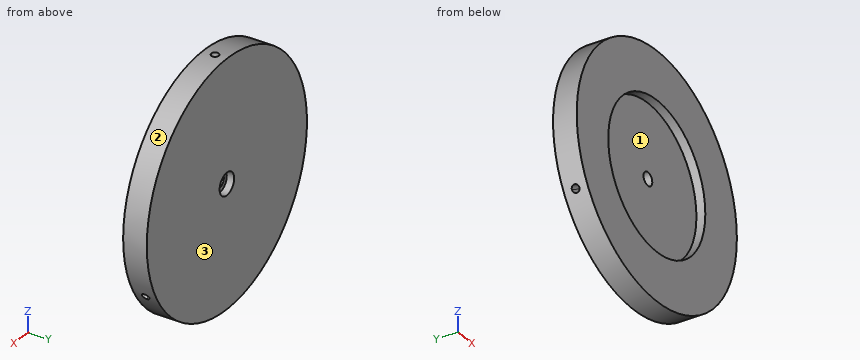
from build123d import *

# Parameters (mm, degrees)
F0_R            = 82.5
F1_DEPTH        = 16
F2_R            = 50
F3_DEPTH        = 6
F6_DEPTH        = 28
F6_COPIES_COUNT = 3
F7_R            = 4.5
F8_DEPTH        = 25
F9_R            = 7.5
F9_R_2          = 4.5
F10_DEPTH       = 5


# Not quite as in the source:
# - a pattern or mirror of a feature is missing from the dataset's text; its kind, count and spacing are read off the source's solid


with BuildPart() as f1:
    # F0 (on Front) → F1 (new body)
    with BuildSketch(Plane.XZ):
        Circle(F0_R)
    extrude(amount=F1_DEPTH)

    # F2 (on face) → F3 (cut)
    with BuildSketch(Plane.XZ.offset(16)):
        Circle(F2_R)
    extrude(amount=-F3_DEPTH, mode=Mode.SUBTRACT)

    # F5 (on offset) → F6 (cut)
    with BuildSketch(Plane.XY.offset(82.5)):
        with BuildLine():
            ThreePointArc((2.5, -8), (1.767766953, -6.232233047), (0, -5.5))
            Line((0, -5.5), (0, -10.5))
            ThreePointArc((0, -10.5), (1.767766953, -9.767766953), (2.5, -8))
        make_face()
        with BuildLine():
            Line((0, -10.5), (0, -5.5))
            ThreePointArc((0, -5.5), (-2.5, -8), (0, -10.5))
        make_face()
    f6 = extrude(amount=-F6_DEPTH, mode=Mode.SUBTRACT)

    # F6_copies: F6 ×3 about axis
    f6_copies_axis = Axis((0, 0, 0), (0, 1, 0))
    for i in range(1, F6_COPIES_COUNT):
        add(f6.rotate(f6_copies_axis, i * 360 / F6_COPIES_COUNT), mode=Mode.SUBTRACT)

    # F7 (on face) → F8 (cut)
    with BuildSketch(Plane.XZ.offset(10)):
        Circle(F7_R)
    extrude(amount=-F8_DEPTH, mode=Mode.SUBTRACT)

    # F9 (on face) → F10 (cut)
    with BuildSketch(Plane(origin=(0, 0, 0), x_dir=(-1, 0, 0), z_dir=(0, 1, 0))):
        Circle(F9_R)
        Circle(F9_R_2, mode=Mode.SUBTRACT)
    extrude(amount=-F10_DEPTH, mode=Mode.SUBTRACT)


solid = f1.part
Read the model definition and answer for the solid it produces. Units are mm, in the model's axes. Face numbers are marked on the shaded views. Round coordinates to 2 decimals unless told otherwise and drop trailing zeros. Order: outer loops, then holes, each group sorted by start corner. A loop starts at its lowest first (then second) coordinate and runs counter-clockwise, first axis right, second up.
1) Flat-ended cylindrical pins translate along their axes: pin 1 (8 mm diameter, centred on x = 38, z = -24, fed in from +Y); pin 2 (8 mm diameter, centred on x = 18, y = -12, fed in from +Z); pin 3 (7.5 mm diameter, centred on x = 2, z = 0.5, fed in from +Y); pin 4 (3 mm diameter, centred on x = 30, y = -12.5, fed in from +Z). Find the tip coordinate at first contact, or state that the pin passes through.
2) Straight lines are drawn through the part: L1, parallel to X at y = -15, z = -1; L2, parallel to Z at x = 0, y = -8.5; L3, parallel to Y at x = -23.5, z = -30.5. For each, find the intervals that lie inside material, in ascending order.
3) The part is cut by section B-B on x = -21. Write down the section's boundary in (y, z), plus the area to 3 significant figures.
4) The part is cut by section A-A on z = 0. Write down the section's boundary in (x, y).
5) The part is cut by section C-C on z = 67. Write down the section's boundary in (x, y), plus the area to 3 significant figures.
6) The part is cut by section D-D on z = 24.5. Write down the section's boundary in (x, y), plus the area to 3 significant figures.
7) The mould has two halves that part along Z. Classify the marked faces 1, 2 and 3: released by +Z, released by -Z, zero draft, split by the parting line, or undercut.
Resolved:
1. pin 1: stops at y = 0
1. pin 2: stops at z = 81.3
1. pin 3: stops at y = -5
1. pin 4: stops at z = 77.42
2. L1: x = -82.49 to -49.99, 49.99 to 82.49
2. L2: z = -82.5 to -4.5, 4.5 to 54.5
2. L3: y = -10 to 0
3. outline: (-16, -79.78) - (0, -79.78) - (0, 79.78) - (-16, 79.78) - (-16, 45.38) - (-10, 45.38) - (-10, -45.38) - (-16, -45.38) - close
3. area: 2,010 mm2
4. outline: (-82.5, -16) - (-50, -16) - (-50, -10) - (-4.5, -10) - (-4.5, -5) - (-7.5, -5) - (-7.5, 0) - (-82.5, 0) - close; (4.5, -10) - (50, -10) - (50, -16) - (82.5, -16) - (82.5, 0) - (7.5, 0) - (7.5, -5) - (4.5, -5) - close
5. outline: (-48.14, -16) - (48.14, -16) - (48.14, 0) - (-48.14, 0) - close; hole circle Ø5 at (0, -8)
5. area: 1,520 mm2
6. outline: (-78.78, -16) - (-43.59, -16) - (-43.59, -10) - (43.59, -10) - (43.59, -16) - (78.78, -16) - (78.78, 0) - (-78.78, 0) - close
6. area: 2,000 mm2
7. face 1: undercut
7. face 2: split by the parting line
7. face 3: zero draft
